Can you work these out from the model? Positions are in its coordinate system, mm. Coordinates: 2 decimals unless noted, no trailing zeros. Write each loop counter-clockwise with the first axis right and the second up, starting at its lowest first coordinate (ties: lowest second). Pieces come first, ordered by that corner, then holes. Notation, with made-up numbers: (57.5, 79.25) -> (108.5, 79.25) arc R11 ccw to (108.5, 97.25) -> close; hole circle Ø4 at (89.25, -34.5). An arc over 180 degrees is marked (long way). Use one line per item in the form item = value.
```python
from build123d import *

# Parameters (mm, degrees)
SKETCH_1_W          = 2.54
SKETCH_1_H          = 2.54
EXTRUDE_1_DEPTH     = 2.54
SKETCH_2_W          = 0.6
SKETCH_2_H          = 0.6
EXTRUDE_2_DEPTH     = 5.6
SKETCH_3_W          = 0.6
SKETCH_3_H          = 0.6
EXTRUDE_3_DEPTH     = 3.2
CHAMFER_1_SIZE      = 0.1
CHAMFER_2_SIZE      = 0.5
SKETCH_4_R          = 0.041822452
CUT_EXTRUDE_1_DEPTH = 10


with BuildPart() as part:
    # 草图1 → 凸台-拉伸1 (new body)
    with BuildSketch(Plane(origin=(0, 0, 0), x_dir=(1, 0, 0), z_dir=(0, 1, 0))):
        Rectangle(SKETCH_1_W, SKETCH_1_H)
    extrude(amount=EXTRUDE_1_DEPTH)

    # 草图2 → 凸台-拉伸2 (add)
    with BuildSketch(Plane(origin=(0, 2.54, 0), x_dir=(1, 0, 0), z_dir=(0, 1, 0))):
        Rectangle(SKETCH_2_W, SKETCH_2_H)
    extrude(amount=EXTRUDE_2_DEPTH)

    # 草图3 → 凸台-拉伸3 (add)
    with BuildSketch(Plane.XZ):
        Rectangle(SKETCH_3_W, SKETCH_3_H)
    extrude(amount=EXTRUDE_3_DEPTH)

    # 倒角1
    chamfer_1_edges = [part.edges().sort_by_distance(p)[0] for p in [
        (0.3, 8.14, 0),
        (0, 8.14, -0.3),
        (-0.3, 8.14, 0),
        (0, 8.14, 0.3),
        (-0.3, -3.2, 0),
        (0, -3.2, -0.3),
        (0.3, -3.2, 0),
        (0, -3.2, 0.3),
    ]]
    chamfer(chamfer_1_edges, length=CHAMFER_1_SIZE)

    # 倒角2
    chamfer_2_edges = [part.edges().sort_by_distance(p)[0] for p in [
        (1.27, 1.27, 1.27),
        (-1.27, 1.27, 1.27),
        (-1.27, 1.27, -1.27),
        (1.27, 1.27, -1.27),
    ]]
    chamfer(chamfer_2_edges, length=CHAMFER_2_SIZE)

    # 草图4 → 切除-拉伸1 (cut)
    with BuildSketch(Plane.XZ.offset(3.2)):
        with Locations(Location((0, 0, 0), (0, 0, 270))):
            Circle(SKETCH_4_R)
    extrude(amount=-CUT_EXTRUDE_1_DEPTH, mode=Mode.SUBTRACT)


solid = part.part
```
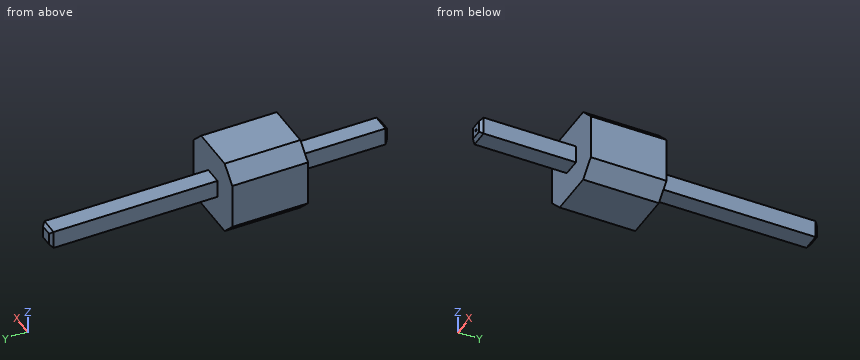
Q1. Suppose I cut it at C-C (x = -0.5). Write out the boundary of the cut face in (y, z), then the cut area to 3 significant figures.
Return value:
outline = (0, -1.27) -> (2.54, -1.27) -> (2.54, 1.27) -> (0, 1.27) -> close
area = 6.45 mm2
Q2. Suppose I cut it at A-A (y = 5.25). Write out the boundary of the cut face in (x, z).
Return value:
outline = (-0.3, -0.3) -> (0.3, -0.3) -> (0.3, 0.3) -> (-0.3, 0.3) -> close; hole circle Ø0.08 at (0, 0)
Q3. Will these pins go through, and if not, where does the flat tip stop? pin 1 (0.7 mm diameter, centred on y = -2, z = 0, fed in from +X); pin 2 (1 mm diameter, centred on x = -1, y = -1.5, fed in from +Z); pin 3 (1 mm diameter, centred on y = 0.5, z = -1, fed in from +X); pin 4 (0.5 mm diameter, centred on x = 0, y = 6, fed in from +Z).
Return value:
pin_1 = 0.3
pin_2 = through
pin_3 = 1.27
pin_4 = 0.3
Q4. Suppose I cut it at B-B (z = -0.9). Write out the boundary of the cut face in (x, y).
Return value:
outline = (-1.14, 0) -> (1.14, 0) -> (1.14, 2.54) -> (-1.14, 2.54) -> close
Q5. If I drill on line 1 (Y direction, x = 0.8, z = -0.1); line 2 (Z direction, x = 0.2, y = 5.5); line 3 (Z direction, x = 0.9, y = 0.25), over which ranges is the centre line in solid material (lowest first)? Write a range as from..to.
Return value:
line_1 = 0..2.54
line_2 = -0.3..0.3
line_3 = -1.14..1.14
